Part model, mm, in its own coordinate system. A direction names the side the tool comes from. Round coordinates to 2 decimals unless told otherwise and drop trailing zeros. Loops run counter-clockwise (first coordinate to the right, second up) from the corner with the lowest first, then second, coordinate; pieces in that order, holes last. Notation, with made-up numbers: (3, -24) -> (19, -24) arc R18 ccw to (19, -19) -> close; hole circle Ø1 at (85.5, 89). An arc over 180 degrees is marked (long way). Answer as CSV lines item,"result".
from build123d import *

# Parameters (mm, degrees)
F1_DEPTH = 20
F2_R     = 1.657373
F3_DEPTH = 4.354743
F4_R     = 1.445676
F5_DEPTH = 5.844262
F6_R     = 2.236419
F7_DEPTH = 30.325829


with BuildPart() as f1:
    # F0 (on Top) → F1 (new body)
    with BuildSketch(Plane.XY):
        with BuildLine():
            ThreePointArc((7.519909, -1.100443), (-7.6, 0), (7.519909, 1.100443))
            Line((7.519909, 1.100443), (19.17907, 1.100443))
            Line((19.17907, 1.100443), (19.17907, 6.944705))
            Line((19.17907, 6.944705), (13.478497, 6.944705))
            ThreePointArc((13.478497, 6.944705), (7.893045, 12.94599), (0, 15.162414))
            Line((0, 15.162414), (-26.202165, 15.162414))
            Line((-26.202165, 15.162414), (-26.202165, 10.25))
            Line((-26.202165, 10.25), (-10.786354, 10.25))
            Line((-10.786354, 10.25), (-10.786354, -10.25))
            Line((-10.786354, -10.25), (-26.202165, -10.25))
            Line((-26.202165, -10.25), (-26.202165, -15.162414))
            Line((-26.202165, -15.162414), (0, -15.162414))
            ThreePointArc((0, -15.162414), (8.578608, -12.502252), (14.147076, -5.455186))
            Line((14.147076, -5.455186), (19.17907, -5.455186))
            Line((19.17907, -5.455186), (19.17907, -1.100443))
            Line((19.17907, -1.100443), (7.519909, -1.100443))
        make_face()
    extrude(amount=F1_DEPTH)

    # F2 (on face) → F3 (cut, through all)
    with BuildSketch(Plane.XZ.offset(5.455186)):
        with Locations((16.663073, 10)):
            Circle(F2_R)
    extrude(amount=-F3_DEPTH, mode=Mode.SUBTRACT)

    # F4 (on face) → F5 (cut, through all)
    with BuildSketch(Plane(origin=(0, 6.944705, 0), x_dir=(-1, 0, 0), z_dir=(0, 1, 0))):
        with Locations((-16.328784, 10)):
            Circle(F4_R)
    extrude(amount=-F5_DEPTH, mode=Mode.SUBTRACT)

    # F6 (on face) → F7 (cut, through all)
    with BuildSketch(Plane.XZ.offset(15.162414)):
        with Locations((-17.060504, 10)):
            Circle(F6_R)
    extrude(amount=-F7_DEPTH, mode=Mode.SUBTRACT)


solid = f1.part
Q1. Saw through at B-B, the plane x = 5.5. Write the cut outline in (y, z) (3 decimals), then the cut area to 3 significant figures.
Geometry results:
outline,"(-14.13, 0) -> (-5.245, 0) -> (-5.245, 20) -> (-14.13, 20) -> close; (5.245, 0) -> (14.13, 0) -> (14.13, 20) -> (5.245, 20) -> close"
area,"355 mm2"
Q2. Two-plate mould, pull along Y, no slides. Class faces 1 (the face through (-13, 15.162, 10)), 2 (the face through (13, -1.1, 10)), 3 (the face through (-15.858, 12.672, 11.886)), 4 (the face through (14.4, -5.455, 9.9)): pulls with the +Y half, pulls with the -Y half, needs draft (parallel to the pull), parting line crosses it, or undercut.
Geometry results:
face 1,"pulls with the +Y half"
face 2,"undercut"
face 3,"needs draft"
face 4,"pulls with the -Y half"
Q3. Saw through at C-C, the plane z = 16. Write the cut outline in (x, y), then the cut area to 3 significant figures.
Geometry results:
outline,"(-26.2, -15.16) -> (0, -15.16) arc R15.16 ccw to (14.15, -5.46) -> (19.18, -5.46) -> (19.18, -1.1) -> (7.52, -1.1) arc R7.6 cw (long way) to (7.52, 1.1) -> (19.18, 1.1) -> (19.18, 6.94) -> (13.48, 6.94) arc R15.16 ccw to (0, 15.16) -> (-26.2, 15.16) -> (-26.2, 10.25) -> (-10.79, 10.25) -> (-10.79, -10.25) -> (-26.2, -10.25) -> close"
area,"688 mm2"
Q4. Drop flat-ended pins along their axis: P1, Ø4, axis at x = -17.06, z = 10, coming from the +Y side; P2, Ø2.5, axis at x = 16.66, z = 10, coming from the -Y side; P3, Ø4, axis at y = 2, z = 11.5, coming from the -X side; P4, Ø2, axis at y = -7.5, z = 5.5, coming from the +X side. Give the stop position or say it passes through.
Geometry results:
P1,"through"
P2,"y = 1.1"
P3,"x = -10.79"
P4,"x = 13.7"
Q5. Saw through at A-A, the plane z = 10. Give the number of separate pieces and of enclosed holes in the cut face, then the cut area to 3 significant figures.
Geometry results:
separate pieces,"5"
enclosed holes,"0"
area,"613 mm2"
Q6. Saw through at D-D, the plane y = -7. Write the cut outline in (x, z).
Geometry results:
outline,"(-10.79, 0) -> (-2.96, 0) -> (-2.96, 20) -> (-10.79, 20) -> close; (2.96, 0) -> (13.45, 0) -> (13.45, 20) -> (2.96, 20) -> close"
Q7. Which spindle directions (+Z, -Z, +X, -X, +Y, -Y) get a long thin tool onto all of the face, cutting with end or side? Do faces 5 (the face through (13, 1.1, 10)), 6 (the face through (-20, 10.25, 10)), 7 (the face through (17.476, 4.063, 9.12)), 8 (the face through (-9, 0, 0)), 9 (the face through (8.473, -12.574, 9.86)). Say none if no direction does.
Geometry results:
face 5,"+Z, -Z, +X"
face 6,"+Z, -Z, -X"
face 7,"+Y"
face 8,"-Z, +X, -X, +Y, -Y"
face 9,"+Z, -Z, +X, -Y"
Q8. Drill centre lines: line 1 along Y through (x, z) = (-19.5, 8.25); line 2 along X through (y, z) = (-5, 11.25); line 3 along X through (y, z) = (-4, 9). Where is each one in solid material? Low to high.
Geometry results:
line 1,"-15.16 to -10.25, 10.25 to 15.16"
line 2,"-10.79 to -5.72, 5.72 to 15.57, 17.75 to 19.18"
line 3,"-10.79 to -6.46, 6.46 to 15.34, 17.98 to 19.18"
